Check sheet for the modelled part. Datum: model origin and axes. Units: mm. A direction names the side the tool comes from. Coordinates: 2 decimals unless noted, no trailing zeros. Write each loop counter-clockwise with the first axis right and the second up, starting at its lowest first coordinate (ties: lowest second). Pieces come first, ordered by that corner, then holes. Notation, with made-up numbers: (8, 17.5) - (26, 17.5) arc R23 ccw to (26, 27.5) - close; hole circle Ø2 at (8, -26.5). An arc over 180 degrees is marked (long way). Write each question's results on one line, items separated by ' | '.
from build123d import *

# Parameters (mm, degrees)
F1_DEPTH = 28
F2_DEPTH = 4
F4_DEPTH = 4
F6_DEPTH = 4
F7_DEPTH = 4
F9_DEPTH = 4


with BuildPart() as f1:
    # F0 (on Front) → F1 (new body)
    with BuildSketch(Plane.XZ):
        Polygon((10, 24), (10, 0), (14, 0), (14, 28), (-14, 28), (-14, 0), (-10, 0), (-10, 24), align=None)
    extrude(amount=F1_DEPTH)

    # F0 (on Front) → F2 (join)
    with BuildSketch(Plane.XZ):
        Polygon((-10, 0), (0, 0), (10, 0), (10, 24), (-10, 24), align=None)
        with BuildLine():
            Line((2.25, 5.5), (0, 5.5))
            Line((0, 5.5), (-2.25, 5.5))
            ThreePointArc((-2.25, 5.5), (-2.957107, 5.792893), (-3.25, 6.5))
            Line((-3.25, 6.5), (-3.25, 15.5))
            ThreePointArc((-3.25, 15.5), (-2.957107, 16.207107), (-2.25, 16.5))
            Line((-2.25, 16.5), (0, 16.5))
            Line((0, 16.5), (2.25, 16.5))
            ThreePointArc((2.25, 16.5), (2.957107, 16.207107), (3.25, 15.5))
            Line((3.25, 15.5), (3.25, 6.5))
            ThreePointArc((3.25, 6.5), (2.957107, 5.792893), (2.25, 5.5))
        make_face(mode=Mode.SUBTRACT)
    extrude(amount=F2_DEPTH)

    # F3 (on face) → F4 (cut)
    with BuildSketch(Plane.YZ.offset(14)):
        Polygon((-4, 0), (-28, 24), (-28, 0), align=None)
    extrude(amount=-F4_DEPTH, mode=Mode.SUBTRACT)

    # F5 (on face) → F6 (cut)
    with BuildSketch(Plane(origin=(-14, 0, 0), x_dir=(0, -1, 0), z_dir=(-1, 0, 0))):
        Polygon((28, 24), (4, 0), (28, 0), align=None)
    extrude(amount=-F6_DEPTH, mode=Mode.SUBTRACT)

    # F0 (on Front) → F7 (cut)
    with BuildSketch(Plane.XZ):
        with BuildLine():
            Line((-2.25, 5.5), (0, 5.5))
            Line((0, 5.5), (2.25, 5.5))
            ThreePointArc((2.25, 5.5), (2.957107, 5.792893), (3.25, 6.5))
            Line((3.25, 6.5), (3.25, 15.5))
            ThreePointArc((3.25, 15.5), (2.957107, 16.207107), (2.25, 16.5))
            Line((2.25, 16.5), (0, 16.5))
            Line((0, 16.5), (-2.25, 16.5))
            ThreePointArc((-2.25, 16.5), (-2.957107, 16.207107), (-3.25, 15.5))
            Line((-3.25, 15.5), (-3.25, 6.5))
            ThreePointArc((-3.25, 6.5), (-2.957107, 5.792893), (-2.25, 5.5))
        make_face()
    extrude(amount=F7_DEPTH, mode=Mode.SUBTRACT)

    # F8 (on face) → F9 (cut)
    with BuildSketch(Plane.XY.offset(28)):
        with BuildLine():
            Line((-3.25, -12.5), (-3.25, -21.5))
            ThreePointArc((-3.25, -21.5), (-2.957107, -22.207107), (-2.25, -22.5))
            Line((-2.25, -22.5), (2.25, -22.5))
            ThreePointArc((2.25, -22.5), (2.957107, -22.207107), (3.25, -21.5))
            Line((3.25, -21.5), (3.25, -12.5))
            ThreePointArc((3.25, -12.5), (2.957107, -11.792893), (2.25, -11.5))
            Line((2.25, -11.5), (-2.25, -11.5))
            ThreePointArc((-2.25, -11.5), (-2.957107, -11.792893), (-3.25, -12.5))
        make_face()
    extrude(amount=-F9_DEPTH, mode=Mode.SUBTRACT)


solid = f1.part
1. Sectioned sample at B-B (z = 11.5). Record the cut outline in (x, y).
Values follow:
outline: (-14, -15.5) - (-10, -15.5) - (-10, -4) - (-3.25, -4) - (-3.25, 0) - (-14, 0) - close; (3.25, -4) - (10, -4) - (10, -15.5) - (14, -15.5) - (14, 0) - (3.25, 0) - close
2. Sectioned sample at A-A (y = -18.5). Record the cut outline in (x, z), then the cut area to 3 significant figures.
Values follow:
outline: (-14, 14.5) - (-10, 14.5) - (-10, 24) - (-3.25, 24) - (-3.25, 28) - (-14, 28) - close; (3.25, 24) - (10, 24) - (10, 14.5) - (14, 14.5) - (14, 28) - (3.25, 28) - close | area: 162 mm^2
3. Material ranges on L1, parallel to X at y = -12.25, z = 18.25; L2, parallel to X at y = -20, z = 26.5; L3, parallel to Z at x = -6.5, y = -18.5, recorded low to high. Write a range as [from, to].
Values follow:
L1: x = [-14, -10], [10, 14] | L2: x = [-14, -3.25], [3.25, 14] | L3: z = [24, 28]
4. Draft check along Z on faces 6 (the cylindrical face through (-2.949, -1.972, 5.785)), 7 (the flat face through (12, -16, 12)), 8 (the flat face through (4, -4, 12)), 9 (the flat face through (0, -2, 16.5)). Enter one of: pulls with the +Z half, pulls with the -Z half, needs draft (parallel to the pull), parting line crosses it, or undercut.
Values follow:
face 6: undercut | face 7: pulls with the -Z half | face 8: needs draft | face 9: undercut
5. Sectioned sample at D-D (y = -3). Record the cut outline in (x, z).
Values follow:
outline: (-14, 0) - (14, 0) - (14, 28) - (-14, 28) - close; hole (-3.25, 6.5) arc R1 ccw to (-2.25, 5.5) - (2.25, 5.5) arc R1 ccw to (3.25, 6.5) - (3.25, 15.5) arc R1 ccw to (2.25, 16.5) - (-2.25, 16.5) arc R1 ccw to (-3.25, 15.5) - close
6. Access from +Z, -Z, +X, -X, +Y, -Y to the whole of each face (thin tool, end or side, straight path). Record for faces 1 (the flat face through (0, -28, 26)), 2 (the flat face through (-12, -16, 12)), 3 (the cylindrical face through (2.949, -22.215, 26.028)), 4 (the cylindrical face through (-2.965, -1.972, 16.199)), 5 (the flat face through (10, -13, 15)).
Values follow:
face 1: +Z, -Z, +X, -X, -Y | face 2: -Z, +X, -X, -Y | face 3: +Z, -Z | face 4: +Y, -Y | face 5: -Z, -Y
7. Sectioned sample at C-C (z = 25). Record the cut outline in (x, y), then the cut area to 3 significant figures.
Values follow:
outline: (-14, -28) - (14, -28) - (14, 0) - (-14, 0) - close; hole (-3.25, -21.5) arc R1 ccw to (-2.25, -22.5) - (2.25, -22.5) arc R1 ccw to (3.25, -21.5) - (3.25, -12.5) arc R1 ccw to (2.25, -11.5) - (-2.25, -11.5) arc R1 ccw to (-3.25, -12.5) - close | area: 713 mm^2
8. Go/stop test with flat-tipped pins: pin 1 (5 mm diameter, centred on x = -5.5, z = 4, fed in from -Y); pin 2 (8 mm diameter, centred on x = 1.5, y = -12, fed in from -Z); pin 3 (6 mm diameter, centred on x = -10, z = 14, fed in from -Y). Record where each tip stops, or that it passes through.
Values follow:
pin 1: stops at y = -4 | pin 2: stops at z = 24 | pin 3: stops at y = -21
